from build123d import *

# Parameters (mm, degrees)
CROQUIS1_W              = 21
CROQUIS1_H              = 21
CROQUIS1_W_2            = 15
CROQUIS1_H_2            = 15
SALIENTE_EXTRUIR1_DEPTH = 70


with BuildPart() as part:
    # Croquis1 → Saliente-Extruir1 (new body)
    with BuildSketch(Plane.XY):
        Rectangle(CROQUIS1_W, CROQUIS1_H)
        Rectangle(CROQUIS1_W_2, CROQUIS1_H_2, mode=Mode.SUBTRACT)
    extrude(amount=SALIENTE_EXTRUIR1_DEPTH)


solid = part.part
Can you work these out from the model? Positions are in its coordinate system, mm. A direction names the side the tool comes from. Coordinates: 2 decimals unless noted, no trailing zeros. Write each loop counter-clockwise with the first axis right and the second up, starting at its lowest first coordinate (ties: lowest second). Pieces come first, ordered by that corner, then holes. Notation, with made-up numbers: (45.25, 55.25) - (72.25, 55.25) arc R17 ccw to (72.25, 60.25) - close; hole circle Ø6 at (62.5, -24.75). An arc over 180 degrees is marked (long way). Return JSON: item names as keys, results as strings. Group by question number.
Item 1: We'd pull the mould along X, two halves only. Please class faces 3 (the face through (0, 10.5, 35)), 4 (the face through (10.5, 0, 35)), 5 (the face through (7.5, 0, 35)): pulls with the +X half, pulls with the -X half, needs draft (parallel to the pull), parting line crosses it, or undercut.
Item 2: I'm going to push a flat-ended pin straight in: pin 1 Ø8 at (x, y) = (-5.5, -1.5) entering from +Z. Where does the tip first touch, or does it pass through?
Item 3: If we section it at A-A (z = 21): Write out the boundary of the cut face in (x, y), then the cut area to 3 significant figures.
Item 4: Please list where this line runs through material, in increasing order: probe 1 along X at (y, z) = (3.5, 24.5).
Item 5: Which directions (+Z, -Z, +X, -X, +Y, -Y) give clear straight access to the entire face, cutting with the end or side of a thin tool? Please do faces 1 (the face through (-10.5, 0, 35)), 2 (the face through (0, -7.5, 35)).
Item 6: If we section it at B-B (y = 6.25): Write out the boundary of the cut face in (x, z).
Return value:
{
 "1": {"face 3": "needs draft", "face 4": "pulls with the +X half", "face 5": "undercut"},
 "2": {"pin 1": "stops at z = 70"},
 "3": {"outline": "(-10.5, -10.5) - (10.5, -10.5) - (10.5, 10.5) - (-10.5, 10.5) - close; hole (-7.5, -7.5) - (7.5, -7.5) - (7.5, 7.5) - (-7.5, 7.5) - close", "area": "216 mm^2"},
 "4": {"probe 1": "x = -10.5 to -7.5, 7.5 to 10.5"},
 "5": {"face 1": "+Z, -Z, -X, +Y, -Y", "face 2": "+Z, -Z"},
 "6": {"outline": "(-10.5, 0) - (-7.5, 0) - (-7.5, 70) - (-10.5, 70) - close; (7.5, 0) - (10.5, 0) - (10.5, 70) - (7.5, 70) - close"}
}
